Input: part model. Units: mm. Frame: model coordinates. A direction names the side the tool comes from. Give positions to 0.01 mm unless a question says otherwise; leave off trailing zeros. Loops run counter-clockwise (first coordinate to the right, second up) from the corner with the lowest first, then second, coordinate; pieces in that order, holes last. Notation, with made-up numbers: M -32.75,27 L 7.25,27 A19 cw 7.25,63 Z; hole C -39.75,-29.75 d11. An arc over 180 degrees is marked long. Answer as a JSON object with one key per item and string values. Group by question number.
```python
from build123d import *

# Parameters (mm, degrees)
ESQUISSE3_R             = 5.25
ENL_V_MAT_EXTRU_1_DEPTH = 46
ESQUISSE4_W             = 24
ESQUISSE4_H             = 26
ENL_V_MAT_EXTRU_2_DEPTH = 46


with BuildPart() as part:
    # Balayage1: sweep along a path in Esquisse1
    with BuildLine(Plane.XY) as balayage1_path:
        Line((0, 0), (347, 0))
        Line((347, 0), (347, 160))
        Line((347, 160), (0, 160))
    # Esquisse2 → Balayage1 (sweep)
    with BuildSketch(Plane(origin=(0, 0, 0), x_dir=(0, 0, -1), z_dir=(1, 0, 0))):
        with BuildLine():
            Line((-12, -15), (12, -15))
            ThreePointArc((12, -15), (14.121320344, -14.121320344), (15, -12))
            Line((15, -12), (15, 12))
            ThreePointArc((15, 12), (14.121320344, 14.121320344), (12, 15))
            Line((12, 15), (-12, 15))
            ThreePointArc((-12, 15), (-14.121320344, 14.121320344), (-15, 12))
            Line((-15, 12), (-15, -12))
            ThreePointArc((-15, -12), (-14.121320344, -14.121320344), (-12, -15))
        make_face()
        with BuildLine():
            Line((-10, -13), (10, -13))
            ThreePointArc((10, -13), (12.121320344, -12.121320344), (13, -10))
            Line((13, -10), (13, 10))
            ThreePointArc((13, 10), (12.121320344, 12.121320344), (10, 13))
            Line((10, 13), (-10, 13))
            ThreePointArc((-10, 13), (-12.121320344, 12.121320344), (-13, 10))
            Line((-13, 10), (-13, -10))
            ThreePointArc((-13, -10), (-12.121320344, -12.121320344), (-10, -13))
        make_face(mode=Mode.SUBTRACT)
    sweep(path=balayage1_path.line, transition=Transition.RIGHT)

    # Esquisse3 → Enlèv. mat.-Extru.1 (cut)
    with BuildSketch(Plane(origin=(362, 0, 0), x_dir=(0, 0, -1), z_dir=(1, 0, 0))):
        with Locations(Location((0, 80, 0), (0, 0, 90))):
            Circle(ESQUISSE3_R)
    extrude(amount=-ENL_V_MAT_EXTRU_1_DEPTH, mode=Mode.SUBTRACT)

    # Esquisse4 → Enlèv. mat.-Extru.2 (cut)
    with BuildSketch(Plane.XY.offset(15)):
        with Locations((347, 80)):
            Rectangle(ESQUISSE4_W, ESQUISSE4_H)
    extrude(amount=-ENL_V_MAT_EXTRU_2_DEPTH, mode=Mode.SUBTRACT)


solid = part.part
```
1. Section D-D (y = 120). Output: boundary loops of the cut face in (x, z), then the cut area to 3 significant figures.
2. Mould query, pull axis Z, two halves, no side actions, for faces 6 (the flat face through (222, 9, -15)), 7 (the flat face through (206, 163, 13)), 8 (the flat face through (222, 151, 15)), 9 (the flat face through (164, 145, 0)). Classes: pulls with the +Z half, pulls with the -Z half, needs draft (parallel to the pull), parting line crosses it, or undercut.
3. Section A-A (x = 92.5). Count the separate pieces of the cut face and the enclosed holes in it, then the cut area to 3 significant figures.
4. Material intervals for L1, parallel to Y at x = 112.5, z = 5; L2, parallel to X at y = 65, z = 10.5; L3, parallel to Z at x = 346, y = 60, sorted ascending.
5. Reachability of faces 1 (the cylindrical face through (361, 85, 1.6)), 2 (the flat face through (334, 81, 7)), 3 (the flat face through (0, 146, 0)), 4 (the flat face through (332, 81, -6)), 5 (the flat face through (165, 147, 0)) from +Z, -Z, +X, -X, +Y, -Y: full face, straight path, thin tool, end or side. Return the list, or none.
6. Section B-B (y = 80). Output: boundary loops of the cut face in (x, z), then the cut area to 3 significant figures.
7. Section C-C (z = 0). Output: boundary loops of the cut face in (x, y), then the cut area to 3 significant figures.
8. First-contact query: P1, Ø1.4, axis at y = 73.5, z = 13.5, coming from the -X side; P2, Ø1.4, axis at x = 341.5, z = 13, coming from the -Y side; P3, Ø23, axis at x = 167.5, y = 21, coming from the -Z side; P4, Ø1.4, axis at x = 350, z = -13, coming from the +Y side. Flat tips, straight axial feed; report the tip coordinate or a pass-through.
Geometry results:
{
 "1": {"outline": "M 332,-12 A3 ccw 335,-15 L 359,-15 A3 ccw 362,-12 L 362,12 A3 ccw 359,15 L 335,15 A3 ccw 332,12 Z; hole M 334,-10 A3 ccw 337,-13 L 357,-13 A3 ccw 360,-10 L 360,10 A3 ccw 357,13 L 337,13 A3 ccw 334,10 Z", "area": "224 mm2"},
 "2": {"face 6": "pulls with the -Z half", "face 7": "undercut", "face 8": "pulls with the +Z half", "face 9": "needs draft"},
 "3": {"separate pieces": "2", "enclosed holes": "2", "area": "448 mm2"},
 "4": {"L1": "-15 to -13, 13 to 15, 145 to 147, 173 to 175", "L2": "332 to 334.04, 359.96 to 362", "L3": "-15 to -13, 13 to 15"},
 "5": {"face 1": "+X, -X", "face 2": "none", "face 3": "+Z, -Z, -X, +Y, -Y", "face 4": "+Z, -Z, -X", "face 5": "-X"},
 "6": {"outline": "M 332,-12 A3 ccw 335,-15 L 335,-12.24 A3 cw 334,-10 L 334,-5.25 L 332,-5.25 Z; M 332,5.25 L 334,5.25 L 334,10 A3 cw 335,12.24 L 335,15 A3 ccw 332,12 Z; M 359,-15 A3 ccw 362,-12 L 362,-5.25 L 360,-5.25 L 360,-10 A3 cw 359,-12.24 Z; M 359,12.24 A3 cw 360,10 L 360,5.25 L 362,5.25 L 362,12 A3 ccw 359,15 Z", "area": "84.1 mm2"},
 "7": {"outline": "M 0,-15 L 362,-15 L 362,74.75 L 360,74.75 L 360,-13 L 0,-13 Z; M 0,13 L 334,13 L 334,74.75 L 332,74.75 L 332,15 L 0,15 Z; M 0,145 L 332,145 L 332,85.25 L 334,85.25 L 334,147 L 0,147 Z; M 0,173 L 360,173 L 360,85.25 L 362,85.25 L 362,175 L 0,175 Z", "area": "3,370 mm2"},
 "8": {"P1": "x = 332.11", "P2": "y = -14.98", "P3": "z = -15", "P4": "y = 174.98"}
}
